Model file for the job. Use its own axes, mm. Face numbers are marked on the shaded views. A direction names the side the tool comes from. Give positions to 0.01 mm unless a question says otherwise; leave off trailing zeros. Write each loop counter-clockwise with the first axis right and the second up, starting at its lowest first coordinate (ties: lowest second). Pieces come first, ordered by that corner, then holes. Notation, with made-up numbers: (17.5, 84) - (58.5, 84) arc R17 ccw to (58.5, 115) - close; hole circle Ø10 at (21, 51.5). An arc over 180 degrees is marked (long way). One line per item, written item: value. Start each with the question number.
(1) Probe L1, parallel to Y at x = -7, z = 4.75; L2, parallel to Y at x = -6, z = 4; L3, parallel to X at y = 10.25, z = 0. List the from-to ranges inside material, lowest first.
(2) Cut at C-C, the plane x = 0. List the corners of the cut face in (y, z).
(3) Mould opens along X. For the marked faces 1, 2 and 3 say: pulls with the +X half, pulls with the -X half, needs draft (parallel to the pull), parting line crosses it, or undercut.
(4) Cut at D-D, the plane x = 16. List the corners of the cut face in (y, z).
(5) 3-axis set-ups, long thin cutter, end or side, ignore diameter. For the marked faces 4, 5 and 6: which of +Z, -Z, +X, -X, +Y, -Y reach the whole face in a straight line?
(6) Cut at B-B, the plane z = -2. List the corners of the cut face in (x, y).
(7) Drop flat-ended pins along their axis: P1, Ø6, axis at y = 3.5, z = 3.5, coming from the +X side; P2, Ø3, axis at y = 17, z = 4.5, coming from the +X side; P3, Ø3, axis at x = -7, y = 8, coming from the -Z side. Give the stop position or say it passes through.
(8) Cut at A-A, the plane y = 8. List the corners of the cut face in (x, z), and give its area (3 significant figures).
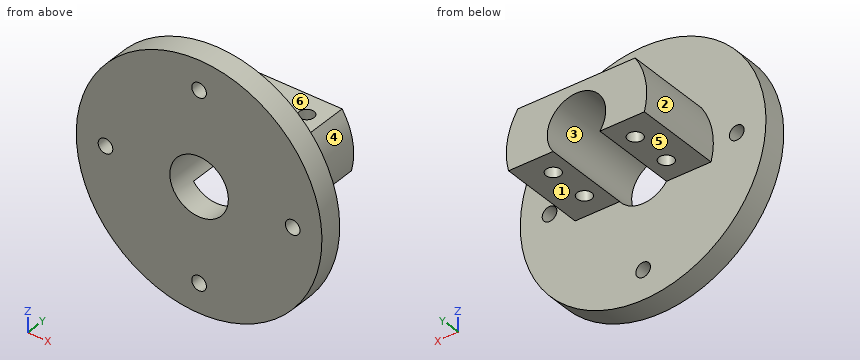
from build123d import *

# Parameters (mm, degrees)
SKETCH_1_R          = 21
EXTRUDE_1_DEPTH     = 4
HOLE_WIZARD_M3_1_D  = 2.5
EXTRUDE_2_DEPTH     = 15
SKETCH_5_R          = 5
CUT_EXTRUDE_1_DEPTH = 36.256205128
HOLE_WIZARD_M3_2_D  = 2.5


with BuildPart() as part:
    # 草图1 → 凸台-拉伸1 (new body)
    with BuildSketch(Plane(origin=(0, 0, 0), x_dir=(1, 0, 0), z_dir=(0, 1, 0))):
        with Locations(Location((0, 0, 0), (0, 0, 270))):
            Circle(SKETCH_1_R)
    extrude(amount=EXTRUDE_1_DEPTH)

    # M3 螺纹孔1 (through all)
    with Locations(Plane(origin=(0, 4, 0), x_dir=(1, 0, 0), z_dir=(0, 1, 0))):
        with Locations((0, 16), (16, 0), (0, -16), (-16, 0)):
            Hole(HOLE_WIZARD_M3_1_D / 2)

    # 草图2 → 凸台-拉伸2 (add)
    with BuildSketch(Plane(origin=(0, 4, 0), x_dir=(1, 0, 0), z_dir=(0, 1, 0))):
        with BuildLine():
            Line((-11.618950039, 3), (11.618950039, 3))
            ThreePointArc((11.618950039, 3), (11.837331556, -1.969157596), (10.021975853, -6.6))
            Line((10.021975853, -6.6), (-10.021975853, -6.6))
            ThreePointArc((-10.021975853, -6.6), (-11.837331556, -1.969157596), (-11.618950039, 3))
        make_face()
    extrude(amount=EXTRUDE_2_DEPTH)

    # 草图5 → 切除-拉伸1 (cut, through all)
    with BuildSketch(Plane(origin=(0, 19, 0), x_dir=(1, 0, 0), z_dir=(0, 1, 0))):
        with Locations(Location((0, 0, 0), (0, 0, 270))):
            Circle(SKETCH_5_R)
    extrude(amount=-CUT_EXTRUDE_1_DEPTH, mode=Mode.SUBTRACT)

    # M3 螺纹孔2 (through all)
    with Locations(Plane(origin=(0, 0, -3), x_dir=(-1, 0, 0), z_dir=(0, 0, -1))):
        with Locations((7, 8), (7, 15), (-7, 8), (-7, 15)):
            Hole(HOLE_WIZARD_M3_2_D / 2)


solid = part.part
Answers follow:
1. L1: y = 0 to 6.75, 9.25 to 13.75, 16.25 to 19
1. L2: y = 0 to 7.25, 8.75 to 14.25, 15.75 to 19
1. L3: x = -12 to -5, 5 to 12
2. outline: (0, -21) - (4, -21) - (4, -17.25) - (0, -17.25) - close; (0, -14.75) - (4, -14.75) - (4, -5) - (0, -5) - close; (0, 5) - (19, 5) - (19, 6.6) - (4, 6.6) - (4, 14.75) - (0, 14.75) - close; (0, 17.25) - (4, 17.25) - (4, 21) - (0, 21) - close
3. face 1: needs draft
3. face 2: pulls with the -X half
3. face 3: undercut
4. outline: (0, -13.6) - (4, -13.6) - (4, -1.25) - (0, -1.25) - close; (0, 1.25) - (4, 1.25) - (4, 13.6) - (0, 13.6) - close
5. face 4: +X, +Y
5. face 5: -Z, +X, -X, +Y
5. face 6: +Z, +X, -X, +Y
6. outline: (-20.9, 0) - (-4.58, 0) - (-4.58, 19) - (-11.83, 19) - (-11.83, 4) - (-20.9, 4) - close; (4.58, 0) - (20.9, 0) - (20.9, 4) - (11.83, 4) - (11.83, 19) - (4.58, 19) - close; hole circle Ø2.5 at (-7, 8); hole circle Ø2.5 at (-7, 15); hole circle Ø2.5 at (7, 8); hole circle Ø2.5 at (7, 15)
7. P1: stops at x = 20.99
7. P2: stops at x = 11.62
7. P3: stops at z = -3
8. outline: (-11.62, -3) - (-8.25, -3) - (-8.25, 6.6) - (-10.02, 6.6) arc R12 ccw to start; (-5.75, -3) - (-4, -3) arc R5 cw (long way) to (4, -3) - (5.75, -3) - (5.75, 6.6) - (-5.75, 6.6) - close; (8.25, -3) - (11.62, -3) arc R12 ccw to (10.02, 6.6) - (8.25, 6.6) - close
8. area: 106 mm²
